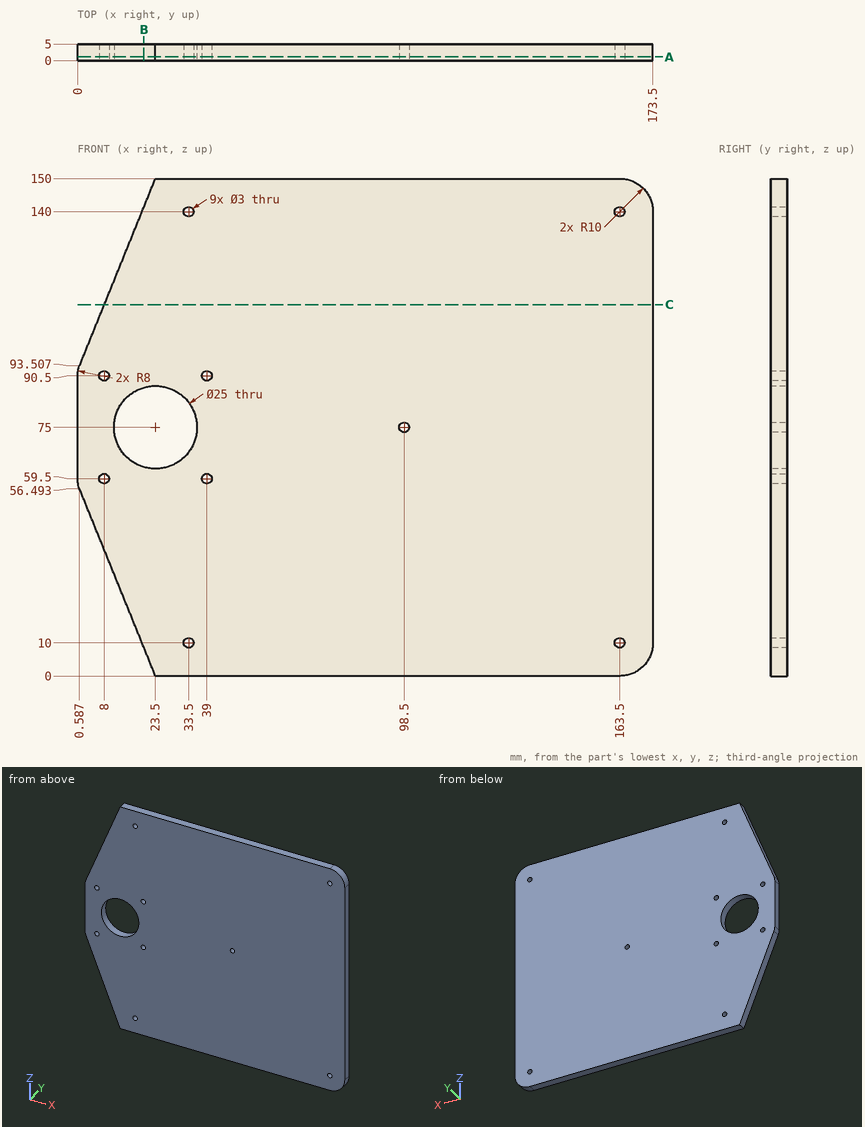
Source: three-view drawing plus pictorial views. Frame: mm from the lowest corner of the part. Give positions to 0.01 mm unless a question says otherwise; leave off trailing zeros. Order: outer loops, then holes, each group sorted by start corner. A loop starts at its lowest first (then second) coordinate and runs counter-clockwise, first axis right, second up. Notation, with made-up numbers: (-8, 24) -> (20, 24) arc R24 cw to (20, 61) -> close; hole circle Ø4 at (65, 17). An arc over 180 degrees is marked (long way). Put each result on its own line as item: value.
Q1. Material intervals for L1, parallel to Z at x = 163.5, y = 3.2; L2, parallel to Z at x = 39, y = 2.4; L3, parallel to X at y = 1.65, z = 90.5, sorted ascending.
Here are the results:
L1: z = 0 to 8.5, 11.5 to 138.5, 141.5 to 150
L2: z = 0 to 58, 61 to 89, 92 to 150
L3: x = 0 to 6.5, 9.5 to 37.5, 40.5 to 173.5
Q2. Section B-B, the plane x = 20. Return loops of the section in (y, z).
Here are the results:
outline: (0, 8.63) -> (5, 8.63) -> (5, 63) -> (0, 63) -> close; (0, 87) -> (5, 87) -> (5, 141.37) -> (0, 141.37) -> close
Q3. Pin query (flat end, axial travel): pin 1 (2.5 mm diameter, centred on x = 8, z = 59.5, fed in from +Y). Return the tip coordinate at first contact, or that it passes through.
Here are the results:
pin 1: passes through
Q4. Section C-C, the plane z = 112. Return loops of the section in (x, y).
Here are the results:
outline: (8.09, 0) -> (173.5, 0) -> (173.5, 5) -> (8.09, 5) -> close
Q5. Section A-A, the plane y = 1.1. Count the separate pieces of the cut face and the enclosed holes in it, then the cut area to 3 significant figures.
Here are the results:
separate pieces: 1
enclosed holes: 10
area: 24,100 mm^2
